Geometry check sheet. Reference: the model listing, model coordinates, mm. A direction names the side the tool comes from. Round coordinates to 2 decimals unless told otherwise and drop trailing zeros. Order: outer loops, then holes, each group sorted by start corner. A loop starts at its lowest first (then second) coordinate and runs counter-clockwise, first axis right, second up.
(1) Draft check along Y on faces 6 (the face through (-13, 22, -27)), 7 (the face through (-31, 6, -24)), 8 (the face through (1.3, 13.1, 27)). Enter one of: pulls with the +Y half, pulls with the -Y half, needs draft (parallel to the pull), parting line crosses it, or undercut.
(2) Thickness scan on L1, parallel to X at y = 14.75, z = 12; L2, parallel to Y at x = 2.5, z = 26.85; L3, parallel to Z at x = 4, y = 17. Record the ranges inside material, lowest first.
(3) Set-up check for faces 1 (the face through (14.5, 11, -27)), 2 (the face through (35.5, 10, 0)), 3 (the face through (-35.5, 11, 0)), 4 (the face through (11, 21, 28)), 5 (the face through (30, 4, -21.5)): record each of +Z, -Z, +X, -X, +Y, -Y from which the full face is reachable in a straight line by a thin tool's end or side.
(4) Cross-section at A-A on z = 5.5. Enter the section's corners in (x, y), and give its area (3 significant figures).
(5) Cross-section at B-B on x = 2.5. Enter the section's corners in (y, z), and give its area (3 significant figures).
(6) Cross-section at D-D on z = -24. Enter the section's corners in (x, y).
(7) Cross-section at C-C on y = 14. Enter the section's corners in (x, z), and give its area (3 significant figures).
(8) Gauge pin test, flat ends, axial feed: P1, Ø2, axis at x = 22.5, z = -18, coming from the +Y side; P2, Ø3.5, axis at x = -3.5, z = 6.5, coming from the +Y side; P3, Ø1, axis at x = 9.5, y = 19, coming from the -Z side. Record the tip position at first contact, or that the pin passes through.
from build123d import *

# Parameters (mm, degrees)
SKETCH1_W           = 71
SKETCH1_H           = 57
BOSS_EXTRUDE1_DEPTH = 3
SKETCH2_W           = 71
SKETCH2_H           = 57
SKETCH2_W_2         = 65
SKETCH2_H_2         = 51
BOSS_EXTRUDE2_DEPTH = 18
SKETCH3_W           = 4
SKETCH3_H           = 4
BOSS_EXTRUDE3_DEPTH = 3
SKETCH4_R           = 3.5
BOSS_EXTRUDE4_DEPTH = 3
CUT_EXTRUDE1_REACH  = 49.932
SKETCH5_R           = 1.4
SKETCH6_W           = 71
SKETCH6_H           = 57
SKETCH6_W_2         = 68
SKETCH6_H_2         = 54
BOSS_EXTRUDE5_DEPTH = 2
SKETCH7_W           = 26
SKETCH7_H           = 2
CUT_EXTRUDE2_DEPTH  = 71.980631161
FILLET1_R           = 1
CUT_EXTRUDE3_REACH  = 72.981
FILLET2_R           = 3
FILLET3_R           = 3
CUT_EXTRUDE4_REACH  = 72.981
SKETCH9_R           = 1.5


with BuildPart() as part:
    # Sketch1 → Boss-Extrude1 (new body)
    with BuildSketch(Plane(origin=(0, 0, 0), x_dir=(1, 0, 0), z_dir=(0, 1, 0))):
        Rectangle(SKETCH1_W, SKETCH1_H)
    extrude(amount=BOSS_EXTRUDE1_DEPTH)

    # Sketch2 → Boss-Extrude2 (add)
    with BuildSketch(Plane(origin=(0, 3, 0), x_dir=(1, 0, 0), z_dir=(0, 1, 0))):
        Rectangle(SKETCH2_W, SKETCH2_H)
        Rectangle(SKETCH2_W_2, SKETCH2_H_2, mode=Mode.SUBTRACT)
    extrude(amount=BOSS_EXTRUDE2_DEPTH)

    # Sketch3 → Boss-Extrude3 (add)
    with BuildSketch(Plane(origin=(0, 3, 0), x_dir=(1, 0, 0), z_dir=(0, 1, 0))):
        with Locations((-30.5, 23.5)):
            Rectangle(SKETCH3_W, SKETCH3_H)
        with Locations((30.5, 23.5)):
            Rectangle(SKETCH3_W, SKETCH3_H)
        with Locations((30.5, -23.5)):
            Rectangle(SKETCH3_W, SKETCH3_H)
        with Locations((-30.5, -23.5)):
            Rectangle(SKETCH3_W, SKETCH3_H)
    extrude(amount=BOSS_EXTRUDE3_DEPTH)

    # Sketch4 → Boss-Extrude4 (add)
    with BuildSketch(Plane(origin=(0, 3, 0), x_dir=(1, 0, 0), z_dir=(0, 1, 0))):
        with Locations(Location((-4.5, -5.5, 0), (0, 0, 270))):
            Circle(SKETCH4_R)
    extrude(amount=BOSS_EXTRUDE4_DEPTH)

    # Sketch5 → Cut-Extrude1 (cut, up to next)
    with BuildSketch(Plane(origin=(0, 6, 0), x_dir=(1, 0, 0), z_dir=(0, 1, 0)), mode=Mode.PRIVATE) as cut_extrude1_sk1:
        with Locations(Location((-4.5, -5.5, 0), (0, 0, 270))):
            Circle(SKETCH5_R)
    cut_extrude1_tool1 = extrude(cut_extrude1_sk1.sketch, amount=-CUT_EXTRUDE1_REACH, mode=Mode.PRIVATE) & part.part
    add(cut_extrude1_tool1.solids().sort_by_distance((-4.5, 6, 5.5))[0], mode=Mode.SUBTRACT)

    # Sketch6 → Boss-Extrude5 (add)
    with BuildSketch(Plane(origin=(0, 21, 0), x_dir=(1, 0, 0), z_dir=(0, 1, 0))):
        Rectangle(SKETCH6_W, SKETCH6_H)
        Rectangle(SKETCH6_W_2, SKETCH6_H_2, mode=Mode.SUBTRACT)
    extrude(amount=BOSS_EXTRUDE5_DEPTH)

    # Sketch7 → Cut-Extrude2 (cut, through all)
    with BuildSketch(Plane.XY.offset(28.5)):
        with Locations((22.5, 22)):
            Rectangle(SKETCH7_W, SKETCH7_H)
    extrude(amount=-CUT_EXTRUDE2_DEPTH, mode=Mode.SUBTRACT)

    # Fillet1
    fillet1_edges = [part.edges().sort_by_distance(p)[0] for p in [
        (9.5, 21, -27.75),
        (9.5, 21, 27.75),
    ]]
    fillet(fillet1_edges, radius=FILLET1_R)
    fillet1_2_edges = [part.edges().sort_by_distance(p)[0] for p in [
        (9.5, 23, -27.75),
        (9.5, 23, 27.75),
    ]]
    fillet(fillet1_2_edges, radius=FILLET1_R - 0.0001)  # a hair under: the kernel refuses the full size

    # Sketch8 → Cut-Extrude3 (cut, up to next)
    with BuildSketch(Plane(origin=(0, 0, -28.5), x_dir=(-1, 0, 0), z_dir=(0, 0, -1)), mode=Mode.PRIVATE) as cut_extrude3_sk1:
        with BuildLine():
            Line((-14.5, 23.871984023), (-8.5, 23.871984023))
            Line((-8.5, 23.871984023), (-8.5, 5))
            ThreePointArc((-8.5, 5), (-9.085786438, 3.585786438), (-10.5, 3))
            Line((-10.5, 3), (-12.5, 3))
            ThreePointArc((-12.5, 3), (-13.914213562, 3.585786438), (-14.5, 5))
            Line((-14.5, 5), (-14.5, 23.871984023))
        make_face()
    cut_extrude3_tool1 = extrude(cut_extrude3_sk1.sketch, amount=-CUT_EXTRUDE3_REACH, mode=Mode.PRIVATE) & part.part
    add(cut_extrude3_tool1.solids().sort_by_distance((11.5, 13.574839, -28.5))[0], mode=Mode.SUBTRACT)

    # Fillet2
    fillet2_edges = [part.edges().sort_by_distance(p)[0] for p in [
        (14.5, 21, -27),
    ]]
    fillet(fillet2_edges, radius=FILLET2_R)

    # Fillet3
    fillet3_edges = [part.edges().sort_by_distance(p)[0] for p in [
        (8.5, 23, -27.75),
    ]]
    fillet(fillet3_edges, radius=FILLET3_R)

    # Sketch9 → Cut-Extrude4 (cut, up to next)
    with BuildSketch(Plane.XY.offset(28.5), mode=Mode.PRIVATE) as cut_extrude4_sk1:
        with Locations((2.5, 14)):
            Circle(SKETCH9_R)
    cut_extrude4_tool1 = extrude(cut_extrude4_sk1.sketch, amount=-CUT_EXTRUDE4_REACH, mode=Mode.PRIVATE) & part.part
    # Sketch9 → Cut-Extrude4 (cut, up to next)
    with BuildSketch(Plane.XY.offset(28.5), mode=Mode.PRIVATE) as cut_extrude4_sk2:
        with Locations((-7.5, 14)):
            Circle(SKETCH9_R)
    cut_extrude4_tool2 = extrude(cut_extrude4_sk2.sketch, amount=-CUT_EXTRUDE4_REACH, mode=Mode.PRIVATE) & part.part
    add(cut_extrude4_tool1.solids().sort_by_distance((2.5, 14, 28.5))[0], mode=Mode.SUBTRACT)
    add(cut_extrude4_tool2.solids().sort_by_distance((-7.5, 14, 28.5))[0], mode=Mode.SUBTRACT)


solid = part.part
Found:
1. face 6: needs draft
1. face 7: pulls with the +Y half
1. face 8: undercut
2. L1: x = -35.5 to -32.5, 32.5 to 35.5
2. L2: y = 0 to 12.5, 15.5 to 21
2. L3: z = -28.5 to -25.5, 25.5 to 28.5
3. face 1: -Z, +Y
3. face 2: +Z, -Z, +X, +Y, -Y
3. face 3: +Z, -Z, -X, +Y, -Y
3. face 4: +X, +Y
3. face 5: +Y
4. outline: (-35.5, 0) - (-5.9, 0) - (-5.9, 6) - (-8, 6) - (-8, 3) - (-32.5, 3) - (-32.5, 21) - (-34, 21) - (-34, 23) - (-35.5, 23) - close; (-3.1, 0) - (35.5, 0) - (35.5, 21) - (32.5, 21) - (32.5, 3) - (-1, 3) - (-1, 6) - (-3.1, 6) - close
4. area: 328 mm2
5. outline: (0, -28.5) - (23, -28.5) - (23, -27) - (21, -27) - (21, -25.5) - (3, -25.5) - (3, 25.5) - (12.5, 25.5) - (12.5, 28.5) - (0, 28.5) - close; (15.5, 25.5) - (21, 25.5) - (21, 27) - (23, 27) - (23, 28.5) - (15.5, 28.5) - close
5. area: 276 mm2
6. outline: (-35.5, 0) - (35.5, 0) - (35.5, 21) - (32.5, 21) - (32.5, 6) - (28.5, 6) - (28.5, 3) - (-28.5, 3) - (-28.5, 6) - (-32.5, 6) - (-32.5, 21) - (-34, 21) - (-34, 23) - (-35.5, 23) - close
7. outline: (-35.5, -28.5) - (8.5, -28.5) - (8.5, -25.5) - (-32.5, -25.5) - (-32.5, 25.5) - (-9, 25.5) - (-9, 28.5) - (-35.5, 28.5) - close; (-6, 25.5) - (1, 25.5) - (1, 28.5) - (-6, 28.5) - close; (4, 25.5) - (32.5, 25.5) - (32.5, -25.5) - (14.5, -25.5) - (14.5, -28.5) - (35.5, -28.5) - (35.5, 28.5) - (4, 28.5) - close
7. area: 696 mm2
8. P1: stops at y = 3
8. P2: stops at y = 6
8. P3: stops at z = 25.5
